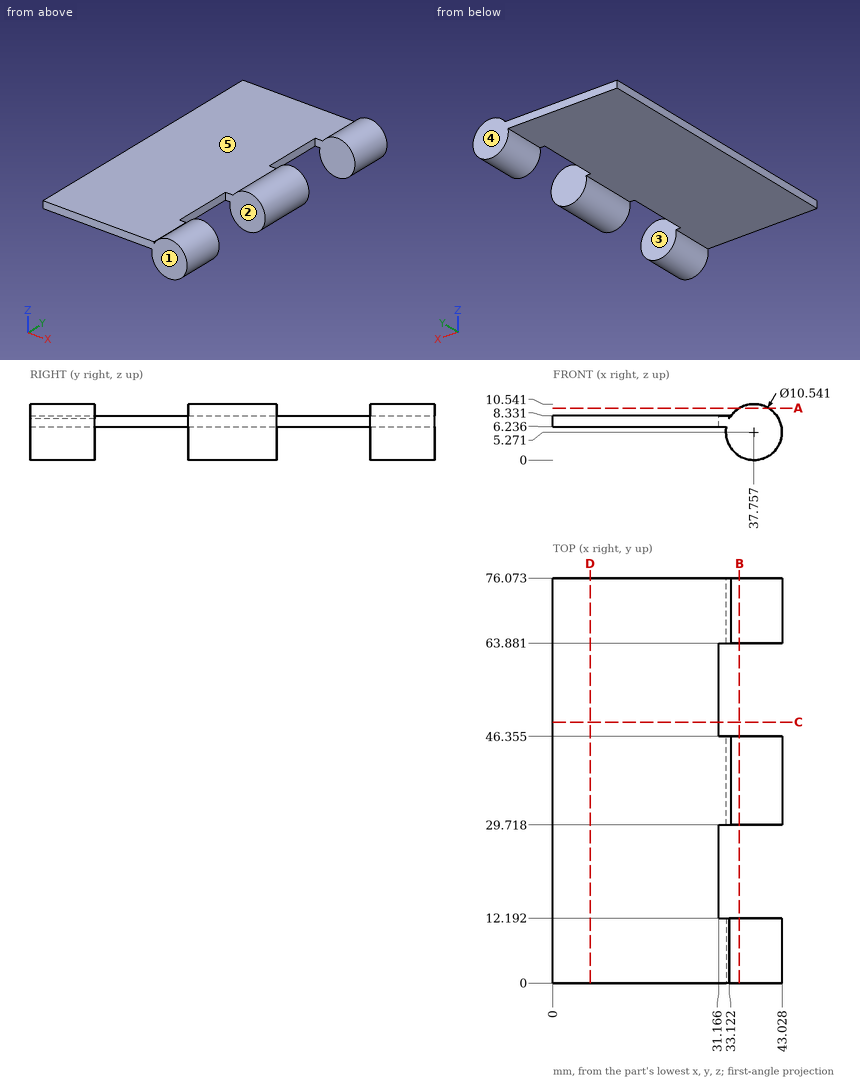
Input: dimensioned drawing with shaded views. Units: mm. Origin: part minimum x, y, z. A direction names the side the tool comes from. Coordinates: 2 decimals unless noted, no trailing zeros. Order: outer loops, then holes, each group sorted by start corner. A loop starts at its lowest first (then second) coordinate and runs counter-clockwise, first axis right, second up.
Item 1: Section query A-A (z = 9.75). Output: boundary loops of the cut face in (x, y) (1 decimal), then the cut area to 3 significant figures.
Answer:
outline: (35, 0) - (40.5, 0) - (40.5, 12.2) - (35, 12.2) - close; (35, 29.7) - (40.5, 29.7) - (40.5, 46.4) - (35, 46.4) - close; (35, 63.9) - (40.5, 63.9) - (40.5, 76.1) - (35, 76.1) - close
area: 228 mm2
Item 2: Section query C-C (y = 49). Output: boundary loops of the cut face in (x, z) (1 decimal).
Answer:
outline: (0, 6.2) - (31.2, 6.2) - (31.2, 8.3) - (0, 8.3) - close
Item 3: Contact query for flat-ended pins moving along their axis: P1, Ø0.6, axis at y = 24, z = 7, coming from the +X side; P2, Ø3, axis at x = 30, y = 12.5, coming from the +Z side; P3, Ø0.6, axis at y = 7, z = 8, coming from the +X side (1 decimal). Output: stop coordinate, or through.
Answer:
P1: stops at x = 31.17
P2: stops at z = 8.33
P3: stops at x = 42.4
Item 4: Section query B-B (x = 35). Output: boundary loops of the cut face in (y, z) (1 decimal).
Answer:
outline: (0, 0.8) - (12.2, 0.8) - (12.2, 9.8) - (0, 9.8) - close; (29.7, 0.8) - (46.4, 0.8) - (46.4, 9.8) - (29.7, 9.8) - close; (63.9, 0.8) - (76.1, 0.8) - (76.1, 9.8) - (63.9, 9.8) - close
Item 5: Material intervals for line 1 along Y through (x, z) = (41, 4) (1 decimal); line 2 along Z through (x, y) = (21.5, 29) (1 decimal); line 3 along X through (y, z) = (48, 6.5) (1 decimal), sorted ascending.
Answer:
line 1: y = 0 to 12.2, 29.7 to 46.4, 63.9 to 76.1
line 2: z = 6.2 to 8.3
line 3: x = 0 to 31.2
Item 6: Section query D-D (x = 7). Output: boundary loops of the cut face in (y, z) (1 decimal).
Answer:
outline: (0, 6.2) - (76.1, 6.2) - (76.1, 8.3) - (0, 8.3) - close
Item 7: Draft query along Y for the marked faces 3, 4 and 5. Return one class per face: released by +Y, released by -Y, zero draft, split by the parting line, or undercut.
Answer:
face 3: undercut
face 4: released by +Y
face 5: zero draft
Item 8: Access query for the marked faces 1 and 2. Directions: +Z, -Z, +X, -X, +Y, -Y. A direction counts if a zero-diameter tool reaches every point of the face in a straight line with its end or side. Return the directions, or none.
Answer:
face 1: +Z, -Z, +X, -X, -Y
face 2: +Z, -Z, +X
